Source: CAD feature listing. Evaluate the final solid. Frame: model axes, mm. Face numbers are marked on the shaded views. A direction names the side the tool comes from. Round coordinates to 2 decimals unless told otherwise and drop trailing zeros. Put each result on its own line as item: value. Start each with the question number.
1. Material intervals for L1, parallel to X at y = 7.5, z = 6.5; L2, parallel to X at y = 11.15, z = 11; L3, parallel to Y at x = -4, z = 46, sorted ascending.
2. Set-up query: the marked faces 1 and 2. Return all of +Z, -Z, +X, -X, +Y, -Y with unobstructed straight access to the full face (end or side cutting, diameter ignored); none if empty.
3. Draft query along X for the marked faces 3 and 4. Return one class per face: pulls with the +X half, pulls with the -X half, needs draft (parallel to the pull), parting line crosses it, or undercut.
4. Contact query for flat-ended pins moving along their axis: pin 1 (6 mm diameter, centred on y = 0, z = 50, fed in from -X); pin 2 (6 mm diameter, centred on y = -8.5, z = 10.5, fed in from -X); pin 3 (2 mm diameter, centred on x = -8.59, z = 11, fed in from +Y); pin 4 (10 mm diameter, centred on x = -14.5, y = 7, fed in from +Z). Output: stop coordinate, or through.
5. Cut plane A-A (z = 11). State how many separate pieces and enclosed holes the cut face has, then the cut area to 3 significant figures.
```python
from build123d import *

# Parameters (mm, degrees)
SKETCH_1_W               = 25
SKETCH_1_H               = 25
EXTRUDE_1_DEPTH          = 60
EXTRUDE_4_DEPTH          = 25
CUT_EXTRUDE_START        = -25
CUT_EXTRUDE_4_DEPTH      = 25
SKETCH_4_W               = 41.211163986
SKETCH_4_H               = 12.5
CUT_EXTRUDE_2_DEPTH      = 19.5
SKETCH_2_R               = 3
CUT_EXTRUDE_1_DEPTH      = 36.406845426
FILLET_1_R               = 2
SKETCH_6_W               = 3.397693812
SKETCH_6_H               = 8.5
SKETCH_6_H_2             = 17
CUT_EXTRUDE_5_DEPTH      = 15
CUT_EXTRUDE_6_DEPTH      = 31
CUT_EXTRUDE_6_DEPTH_BACK = 10
SKETCH_7_R               = 1.25
FILLET_2_R               = 2


# Read off the part's stored shape, not the designer's step: 컷-돌출4
with BuildPart() as part:
    # 스케치1 → 보스-돌출1 (new body)
    with BuildSketch(Plane.XY):
        Rectangle(SKETCH_1_W, SKETCH_1_H)
    extrude(amount=EXTRUDE_1_DEPTH)

    # 스케치5 → 보스-돌출4 (add)
    with BuildSketch(Plane(origin=(0, 12.5, 0), x_dir=(1, 0, 0), z_dir=(0, 1, 0))):
        with BuildLine():
            add(Edge.make_bspline(
                [(2.878979614, 0), (12.5, -24.697131942), (12.5, -60)],
                knots=[0, 0, 0, 1, 1, 1], degree=2))
            Line((2.878979614, 0), (-12.5, 0))
            Line((-12.5, 0), (-12.5, -60))
            Line((-12.5, -60), (12.5, -60))
        make_face()
        with BuildLine():
            Line((-12.5, -60), (-12.5, 0))
            add(Edge.make_bspline(
                [(-12.5, 0), (-25.857752506, -24.697131942), (-12.5, -60)],
                knots=[0, 0, 0, 1, 1, 1], degree=2))
        make_face()
    extrude(amount=-EXTRUDE_4_DEPTH)

    # 컷-돌출4 outline → 컷-돌출4 (cut)
    with BuildSketch(Plane(origin=(0, 12.5, 0), x_dir=(1, 0, 0), z_dir=(0, 1, 0)).offset(CUT_EXTRUDE_START)):
        with BuildLine():
            Line((12.5, 0), (2.878979614, 0))
            add(Edge.make_bspline(
                [(2.878979614, 0), (12.5, -24.697131942), (12.5, -60)],
                knots=[0, 0, 0, 1, 1, 1], degree=2))
            Line((12.5, -60), (12.5, 0))
        make_face()
    extrude(amount=CUT_EXTRUDE_4_DEPTH, mode=Mode.SUBTRACT)

    # 스케치4 → 컷-돌출2 (cut)
    with BuildSketch(Plane.XY.offset(60)):
        with Locations((-1.817465194, 6.25)):
            Rectangle(SKETCH_4_W, SKETCH_4_H)
    extrude(amount=-CUT_EXTRUDE_2_DEPTH, mode=Mode.SUBTRACT)

    # 스케치2 → 컷-돌출1 (cut)
    with BuildSketch(Plane(origin=(0, 12.5, 0), x_dir=(1, 0, 0), z_dir=(0, 1, 0))):
        with Locations(Location((0, -51, 0), (0, 0, 270))):
            Circle(SKETCH_2_R)
    extrude(amount=-CUT_EXTRUDE_1_DEPTH, mode=Mode.SUBTRACT)

    # 필렛1
    fillet_1_edges = [part.edges().sort_by_distance(p)[0] for p in [
        (2.878979614, 0, 0),
        (-12.5, 0, 0),
    ]]
    fillet(fillet_1_edges, radius=FILLET_1_R)

    # 스케치6 → 컷-돌출5 (cut)
    with BuildSketch(Plane(origin=(0, 0, 0), x_dir=(-1, 0, 0), z_dir=(0, 0, -1))):
        with Locations((1.196360316, 4.25)):
            Rectangle(SKETCH_6_W, SKETCH_6_H)
        with Locations((1.196360316, -4.25)):
            Rectangle(SKETCH_6_W, SKETCH_6_H)
        with Locations((8.594054128, 0)):
            Rectangle(SKETCH_6_W, SKETCH_6_H_2)
    extrude(amount=-CUT_EXTRUDE_5_DEPTH, mode=Mode.SUBTRACT)

    # 스케치7 → 컷-돌출6 (cut, two sides: drawn at the far end of the back side and taken through both)
    with BuildSketch(Plane.XZ.offset(-8.5).offset(-CUT_EXTRUDE_6_DEPTH_BACK)):
        with Locations(Location((-1.196360316, 4, 0), (0, 0, 90))):
            Circle(SKETCH_7_R)
        with Locations(Location((-1.196360316, 11, 0), (0, 0, 90))):
            Circle(SKETCH_7_R)
        with Locations(Location((-8.594054128, 4, 0), (0, 0, 90))):
            Circle(SKETCH_7_R)
        with Locations(Location((-8.594054128, 11, 0), (0, 0, 90))):
            Circle(SKETCH_7_R)
    extrude(amount=CUT_EXTRUDE_6_DEPTH + CUT_EXTRUDE_6_DEPTH_BACK, mode=Mode.SUBTRACT)

    # 필렛2
    fillet_2_edges = [part.edges().sort_by_distance(p)[0] for p in [
        (12.5, -6.25, 60),
    ]]
    fillet(fillet_2_edges, radius=FILLET_2_R)


solid = part.part
```
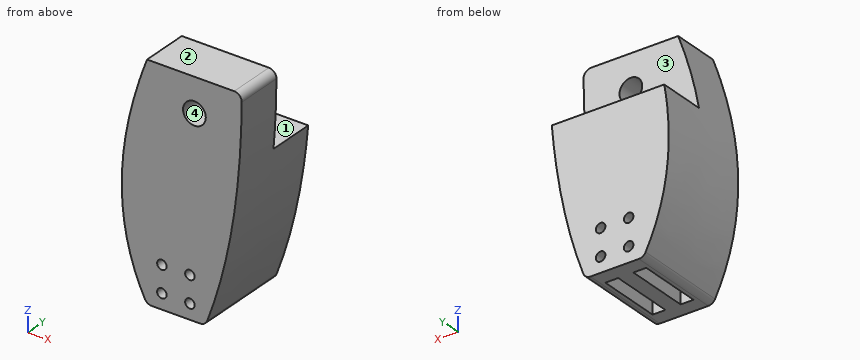
Solution:
1. L1: x = -15.48 to -10.29, -6.9 to -2.9, 0.5 to 5.19
1. L2: x = -16.98 to -9.84, -7.34 to -2.45, 0.05 to 6.54
1. L3: y = -12.5 to 0
2. face 1: +Z, +X, -X, +Y
2. face 2: +Z, +X, -X, +Y, -Y
3. face 3: needs draft
3. face 4: undercut
4. pin 1: stops at x = -16.6
4. pin 2: stops at x = -17.63
4. pin 3: passes through
4. pin 4: stops at z = 40.5
5. separate pieces: 3
5. enclosed holes: 0
5. area: 432 mm^2
